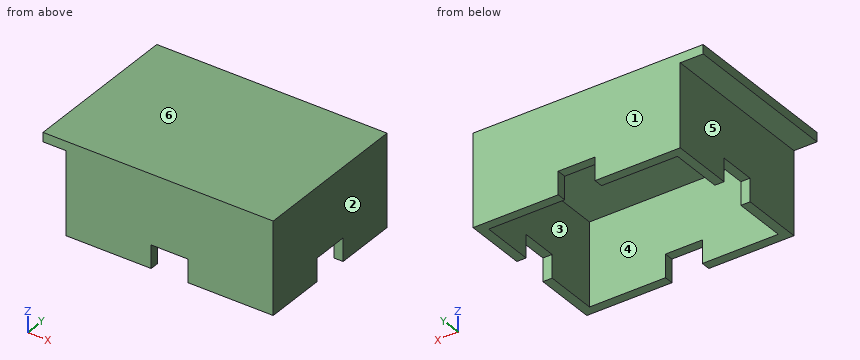
from build123d import *

# Parameters (mm, degrees)
BOX006_W     = 2
BOX006_H     = 8
BOX006_DEPTH = 5
BOX005_W     = 2
BOX005_H     = 8
BOX005_DEPTH = 5
BOX004_W     = 8
BOX004_H     = 2
BOX004_DEPTH = 5
BOX003_W     = 8
BOX003_H     = 2
BOX003_DEPTH = 5
BOX002_W     = 41
BOX002_H     = 31
BOX002_DEPTH = 18
BOX001_W     = 5
BOX001_H     = 35
BOX001_DEPTH = 18
BOX_W        = 50
BOX_H        = 35
BOX_DEPTH    = 20


with BuildPart() as cubo006:
    # Box006 → Box006 (new body)
    with BuildSketch(Plane(origin=(48, 13.5, 0), x_dir=(1, 0, 0), z_dir=(0, 0, 1))):
        with Locations((1, 4)):
            Rectangle(BOX006_W, BOX006_H)
    extrude(amount=BOX006_DEPTH)


with BuildPart() as cubo005:
    # Box005 → Box005 (new body)
    with BuildSketch(Plane(origin=(5, 13.5, 0), x_dir=(1, 0, 0), z_dir=(0, 0, 1))):
        with Locations((1, 4)):
            Rectangle(BOX005_W, BOX005_H)
    extrude(amount=BOX005_DEPTH)


with BuildPart() as cubo004:
    # Box004 → Box004 (new body)
    with BuildSketch(Plane(origin=(23.5, 33, 0), x_dir=(1, 0, 0), z_dir=(0, 0, 1))):
        with Locations((4, 1)):
            Rectangle(BOX004_W, BOX004_H)
    extrude(amount=BOX004_DEPTH)


with BuildPart() as cubo003:
    # Box003 → Box003 (new body)
    with BuildSketch(Plane(origin=(23.5, 0, 0), x_dir=(1, 0, 0), z_dir=(0, 0, 1))):
        with Locations((4, 1)):
            Rectangle(BOX003_W, BOX003_H)
    extrude(amount=BOX003_DEPTH)


with BuildPart() as cubo002:
    # Box002 → Box002 (new body)
    with BuildSketch(Plane(origin=(7, 2, 0), x_dir=(1, 0, 0), z_dir=(0, 0, 1))):
        with Locations((20.5, 15.5)):
            Rectangle(BOX002_W, BOX002_H)
    extrude(amount=BOX002_DEPTH)


with BuildPart() as cubo001:
    # Box001 → Box001 (new body)
    with BuildSketch(Plane.XY):
        with Locations((2.5, 17.5)):
            Rectangle(BOX001_W, BOX001_H)
    extrude(amount=BOX001_DEPTH)


with BuildPart() as cut005:
    # Box → Box (new body)
    with BuildSketch(Plane.XY):
        with Locations((25, 17.5)):
            Rectangle(BOX_W, BOX_H)
    extrude(amount=BOX_DEPTH)

    # Cut: cut Cubo001
    add(cubo001.part, mode=Mode.SUBTRACT)

    # Cut001: cut Cubo002
    add(cubo002.part, mode=Mode.SUBTRACT)

    # Cut002: cut Cubo003
    add(cubo003.part, mode=Mode.SUBTRACT)

    # Cut003: cut Cubo004
    add(cubo004.part, mode=Mode.SUBTRACT)

    # Cut004: cut Cubo005
    add(cubo005.part, mode=Mode.SUBTRACT)

    # Cut005: cut Cubo006
    add(cubo006.part, mode=Mode.SUBTRACT)


solid = cut005.part
Source: CAD feature listing. Evaluate the final solid. Frame: model axes, mm. Face numbers are marked on the shaded views. A direction names the side the tool comes from. Round coordinates to 2 decimals unless told otherwise and drop trailing zeros. Order: outer loops, then holes, each group sorted by start corner. A loop starts at its lowest first (then second) coordinate and runs counter-clockwise, first axis right, second up. Notation, with made-up numbers: (53.25, -25.5) - (81.25, -25.5) arc R14 cw to (81.25, -12.5) - close; hole circle Ø4 at (-38, -14). An arc over 180 degrees is marked (long way). Use a Markdown table: item, result. Add a question column.
1. Section query A-A (z = 4.25). Return the cut outline in (x, y).
2. Set-up query: the marked faces 4, 5 and 6. Return all of +Z, -Z, +X, -X, +Y, -Y with unobstructed straight access to the full face (end or side cutting, diameter ignored); none if empty.
3. First-contact query: pin 1 (0.6 mm diameter, centred on x = 48.5, y = 15.5, fed in from -Z); pin 2 (1.5 mm diameter, centred on x = 34.5, y = 20.5, fed in from -Z); pin 3 (2 mm diameter, centred on y = 1, z = 3, fed in from -X); pin 4 (6 mm diameter, centred on x = 8, y = 6, fed in from -Z). Flat tips, straight axial feed; report the tip coordinate or a pass-through.
4. Section query C-C (z = 17). Return the cut outline in (x, y).
5. Section query D-D (x = 40). Return the cut outline in (y, z).
6. Mould query, pull axis X, two halves, no side actions, for the marked faces 1, 2 and 3. Classes: +X half, -X half, draft (parallel to the pull), parting line (faces both ways), or undercut.
7. Line query: probe 1 along X at (y, z) = (11, 5.5); probe 2 along Y at (x, z) = (19, 15); probe 3 along Z at (x, y) = (33.5, 12). Output: solid intervals per line, ascending.
8. Section query B-B (y = 19). Return the cut outline in (x, z), then the cut area to 3 significant figures.
Derived:
| question | item | result |
|---|---|---|
| 1 | outline | (5, 0) - (23.5, 0) - (23.5, 2) - (7, 2) - (7, 13.5) - (5, 13.5) - close; (5, 21.5) - (7, 21.5) - (7, 33) - (23.5, 33) - (23.5, 35) - (5, 35) - close; (31.5, 0) - (50, 0) - (50, 13.5) - (48, 13.5) - (48, 2) - (31.5, 2) - close; (31.5, 33) - (48, 33) - (48, 21.5) - (50, 21.5) - (50, 35) - (31.5, 35) - close |
| 2 | face 4 | -Z |
| 2 | face 5 | -Z, -X, +Y, -Y |
| 2 | face 6 | +Z, +X, -X, +Y, -Y |
| 3 | pin 1 | z = 5 |
| 3 | pin 2 | z = 18 |
| 3 | pin 3 | x = 5 |
| 3 | pin 4 | z = 0 |
| 4 | outline | (5, 0) - (50, 0) - (50, 35) - (5, 35) - close; hole (7, 2) - (48, 2) - (48, 33) - (7, 33) - close |
| 5 | outline | (0, 0) - (2, 0) - (2, 18) - (33, 18) - (33, 0) - (35, 0) - (35, 20) - (0, 20) - close |
| 6 | face 1 | draft |
| 6 | face 2 | +X half |
| 6 | face 3 | undercut |
| 7 | probe 1 | 5 to 7, 48 to 50 |
| 7 | probe 2 | 0 to 2, 33 to 35 |
| 7 | probe 3 | 18 to 20 |
| 8 | outline | (0, 18) - (5, 18) - (5, 5) - (7, 5) - (7, 18) - (48, 18) - (48, 5) - (50, 5) - (50, 20) - (0, 20) - close |
| 8 | area | 152 mm2 |
